```python
from build123d import *

# Parameters (mm, degrees)
SKETCH1_R           = 1.42
BOSS_EXTRUDE1_DEPTH = 10


with BuildPart() as part:
    # Sketch1 → Boss-Extrude1 (new body)
    with BuildSketch(Plane.XY):
        Polygon((109, 80), (109, 77), (115.58, 77), (115.58, 74), (113.33, 74), (113.33, 71.61), (115.58, 71.61), (115.58, 67.61), (118.42, 67.61), (118.42, 71.61), (120.67, 71.61), (120.67, 74), (118.42, 74), (118.42, 77), (125, 77), (125, 80), (143.417515172, 80), (143.417515172, 60), (143.417515172, 20), (143.417515172, 0), (125, 0), (125, 3), (118.42, 3), (118.42, 6), (120.67, 6), (120.67, 8.39), (118.42, 8.39), (118.42, 12.39), (115.58, 12.39), (115.58, 8.39), (113.33, 8.39), (113.33, 6), (115.58, 6), (115.58, 3), (109, 3), (109, 0), (104.593570259, 0), (104.593570259, -12), (58.593570259, -12), (58.593570259, 0), (54.187140517, 0), (54.187140517, 3), (47.607140517, 3), (47.607140517, 6), (49.857140517, 6), (49.857140517, 8.39), (47.607140517, 8.39), (47.607140517, 12.39), (44.767140517, 12.39), (44.767140517, 8.39), (42.517140517, 8.39), (42.517140517, 6), (44.767140517, 6), (44.767140517, 3), (38.187140517, 3), (38.187140517, 0), (0, 0), (-15.602079829, 0), (-15.602079829, 80), (5, 80), (38.187140517, 80), (38.187140517, 77), (44.767140517, 77), (44.767140517, 74), (42.517140517, 74), (42.517140517, 71.61), (44.767140517, 71.61), (44.767140517, 67.61), (47.607140517, 67.61), (47.607140517, 71.61), (49.857140517, 71.61), (49.857140517, 74), (47.607140517, 74), (47.607140517, 77), (54.187140517, 77), (54.187140517, 80), (58.593570259, 80), (58.593570259, 92), (104.593570259, 92), (104.593570259, 80), align=None)
        with Locations((2.037759908, 40)):
            Circle(SKETCH1_R, mode=Mode.SUBTRACT)
        with Locations((2.037759908, 65)):
            Circle(SKETCH1_R, mode=Mode.SUBTRACT)
        with Locations((2.037759908, 15)):
            Circle(SKETCH1_R, mode=Mode.SUBTRACT)
        with Locations((66.593570259, 86)):
            Circle(SKETCH1_R, mode=Mode.SUBTRACT)
        with Locations((96.593570259, 86)):
            Circle(SKETCH1_R, mode=Mode.SUBTRACT)
        with Locations((96.593570259, -6)):
            Circle(SKETCH1_R, mode=Mode.SUBTRACT)
        with Locations((66.593570259, -6)):
            Circle(SKETCH1_R, mode=Mode.SUBTRACT)
        with Locations((-9.374764666, 45)):
            Circle(SKETCH1_R, mode=Mode.SUBTRACT)
        with Locations((-9.374764666, 35)):
            Circle(SKETCH1_R, mode=Mode.SUBTRACT)
        Polygon((136.600558962, 60), (136.600558962, 20), (97.442765105, 20), (97.442765105, 13), (66.593570259, 13), (66.593570259, 20), (23.079003763, 20), (23.079003763, 60), (66.593570259, 60), (66.593570259, 67), (97.442765105, 67), (97.442765105, 60), align=None, mode=Mode.SUBTRACT)
    extrude(amount=BOSS_EXTRUDE1_DEPTH)


solid = part.part
```
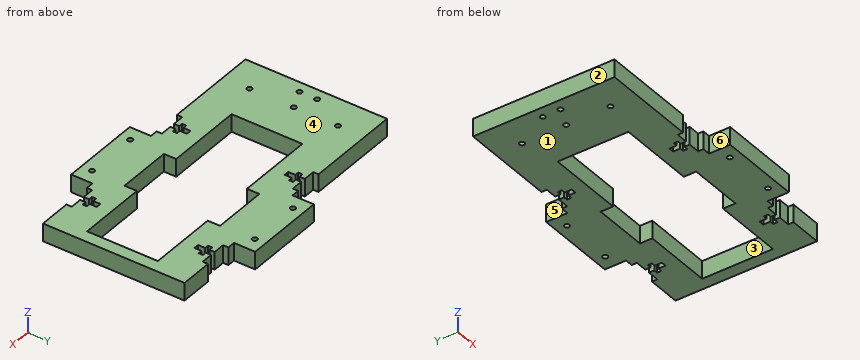
Could you check a few things on this model? Use its own coordinates, in mm. Face numbers are marked on the shaded views. A direction names the side the tool comes from. Round coordinates to 2 decimals unless told otherwise and drop trailing zeros. Write each loop counter-clockwise with the first axis right and the second up, starting at its lowest first coordinate (ties: lowest second). Pieces come first, ordered by that corner, then holes.
(1) Suppose I cut it at D-D on x = 7.5. Write out the boundary of the cut face in (y, z), and give its area (3 significant figures).
Findings below:
outline: (0, 0) - (80, 0) - (80, 10) - (0, 10) - close
area: 800 mm2
(2) Suppose I cut it at A-A on y = 62. Write out the boundary of the cut face in (x, z), and give its area (3 significant figures).
Findings below:
outline: (-15.6, 0) - (66.59, 0) - (66.59, 10) - (-15.6, 10) - close; (97.44, 0) - (143.42, 0) - (143.42, 10) - (97.44, 10) - close
area: 1,280 mm2
(3) For pin 1 (2.5 mm diameter, centred on x = -9.37, y = 45, fed in from +Z); pin 2 (1.1 mm diameter, centred on x = 115, z = 5, fed in from -Y); pin 3 (6 mm diameter, centred on x = 1.5, z = 1.5, fed in from +Y), each with a flat end and sliding along its axis, tell me the tip position at first contact or that it passes through.
Findings below:
pin 1: passes through
pin 2: stops at y = 3
pin 3: stops at y = 80
(4) Suppose I cut it at B-B on x = 89.5. Write out the boundary of the cut face in (y, z).
Findings below:
outline: (-12, 0) - (13, 0) - (13, 10) - (-12, 10) - close; (67, 0) - (92, 0) - (92, 10) - (67, 10) - close
(5) Suppose I cut it at C-C on z = 6.5. State how many separate pieces and enclosed holes the cut face has, and give its area (3 significant figures).
Findings below:
separate pieces: 1
enclosed holes: 10
area: 8,450 mm2
(6) If I drill on probe 1 along X at (y, z) = (71, 6.5); probe 2 along X at (y, z) = (86, 7); probe 3 along Y at (x, z) = (90, 9.75), over which ranges is the centre line in solid material (lowest first)?
Findings below:
probe 1: x = -15.6 to 44.77, 47.61 to 115.58, 118.42 to 143.42
probe 2: x = 58.59 to 65.17, 68.01 to 95.17, 98.01 to 104.59
probe 3: y = -12 to 13, 67 to 92
(7) Thinking about a two-plate mould opening in X: for the marked faces 1, 2 and 3, which applies, +X half, -X half, draft (parallel to the pull), parting line (faces both ways), or undercut?
Findings below:
face 1: draft
face 2: -X half
face 3: undercut
(8) Which directions (+Z, -Z, +X, -X, +Y, -Y) give clear straight access to the entire face, cutting with the end or side of a thin tool? Please do the marked faces 4, 5 and 6.
Findings below:
face 4: +Z, +X, -X, +Y, -Y
face 5: +Z, -Z, -X, +Y
face 6: +Z, -Z, -X, -Y
